from build123d import *

# Parameters (mm, degrees)
BOSS_EXTRUDE4_DEPTH = 4
CUT_EXTRUDE7_DEPTH  = 5
LPATTERN2_COUNT     = 13
LPATTERN2_PITCH     = 9.7389
SKETCH10_W          = 14
SKETCH10_H          = 2.5
BOSS_EXTRUDE5_DEPTH = 115
SKETCH11_R          = 2.5
CUT_EXTRUDE8_DEPTH  = 13


with BuildPart() as part:
    # Sketch9 → Boss-Extrude4 (new body, symmetric)
    with BuildSketch(Plane.XY):
        Polygon((57.5, 6), (49.449989311, 6), (52.64, -0.841), (54.309989311, -0.841), align=None)
        Polygon((52.64, -0.841), (49.449989311, 6), (-57.5, 6), (-57.5, -6), (57.5, -6), (57.5, 6), (54.309989311, -0.841), align=None)
    extrude(amount=BOSS_EXTRUDE4_DEPTH, both=True)

    # Sketch9<4> → Cut-Extrude7 (cut, symmetric)
    with BuildSketch(Plane.XY):
        Polygon((57.5, 6), (49.449989311, 6), (52.64, -0.841), (54.309989311, -0.841), align=None)
    cut_extrude7 = extrude(amount=CUT_EXTRUDE7_DEPTH, both=True, mode=Mode.SUBTRACT)

    # LPattern2: Cut-Extrude7 ×13
    with Locations(*[(-i * LPATTERN2_PITCH, 0, 0) for i in range(1, LPATTERN2_COUNT)]):
        add(cut_extrude7, mode=Mode.SUBTRACT)

    # Sketch10 → Boss-Extrude5 (add)
    with BuildSketch(Plane.ZY.offset(57.5)):
        with Locations((0, -4.75)):
            Rectangle(SKETCH10_W, SKETCH10_H)
    extrude(amount=-BOSS_EXTRUDE5_DEPTH)

    # Sketch11 → Cut-Extrude8 (cut, through all)
    with BuildSketch(Plane.XZ.offset(6)):
        with Locations((-52.5, 0)):
            Circle(SKETCH11_R)
    extrude(amount=-CUT_EXTRUDE8_DEPTH, mode=Mode.SUBTRACT)


solid = part.part
Check sheet for the modelled part. Datum: model origin and axes. Units: mm. A direction names the side the tool comes from. Round coordinates to 2 decimals unless told otherwise and drop trailing zeros. Loops run counter-clockwise (first coordinate to the right, second up) from the corner with the lowest first, then second, coordinate; pieces in that order, holes last. Notation, with made-up numbers: (58.25, 64.5) - (96.25, 64.5) arc R23 ccw to (96.25, 98.5) - close; hole circle Ø8 at (82, 34). An arc over 180 degrees is marked (long way). Answer as CSV lines item,"result". Start each with the question number.
Item 1: Scan lines: line 1 (X direction, y = -1.5, z = 0); line 2 (X direction, y = -1.5, z = 1.5); line 3 (Z direction, x = 51, y = 0.25). Record each from-to range of solid material in increasing order. Write a range as [from, to].
Item 2: Section check A-A (y = 2.25). Count the separate pieces of the cut face and the enclosed holes in it, and give its area (3 significant figures).
Item 3: Section check B-B (x = -42). Record the boundary of the cut face in (y, z).
Item 4: Depth check by flat-ended pin: P1, Ø0.5, axis at x = 53, z = 1.5, coming from the +Y side; P2, Ø6, axis at x = -24.5, z = -1, coming from the +Y side; P3, Ø5, axis at x = 34.5, y = 2, coming from the -Z side; P4, Ø4, axis at x = -52.5, z = 0, coming from the -Y side. Enter the tip coordinate at first touch or a pass-through.
Item 5: Section check C-C (z = 5.25). Record the boundary of the cut face in (x, y).
Item 6: Set-up check for faces 4 (the flat face through (-1, -5, -7)), 5 (the flat face through (-1, 0, -4)), 6 (the flat face through (-26.89, 2.63, 0.06)): record each of +Z, -Z, +X, -X, +Y, -Y from which the full face is reachable in a straight line by a thin tool's end or side.
Item 7: Release check for a two-part mould opening along X. For faces 1 (the flat face through (-1, -5, 7)), 2 (the flat face through (57.5, -1, 0)), 3 (the flat face through (21.806, 2.627, 0.056)) record: +X half, -X half, draft (parallel to the pull), parting line (faces both ways), or undercut.
Report:
1,line 1,"x = [-57.5, -55], [-50, 57.5]"
1,line 2,"x = [-57.5, -54.5], [-50.5, 57.5]"
1,line 3,"z = [-4, 4]"
2,separate pieces,"13"
2,enclosed holes,"0"
2,area,"479 mm2"
3,outline,"(-6, -7) - (-3.5, -7) - (-3.5, -4) - (1.47, -4) - (1.47, 4) - (-3.5, 4) - (-3.5, 7) - (-6, 7) - close"
4,P1,"stops at y = -0.84"
4,P2,"stops at y = 3.94"
4,P3,"stops at z = -4"
4,P4,"passes through"
5,outline,"(-57.5, -6) - (57.5, -6) - (57.5, -3.5) - (-57.5, -3.5) - close"
6,face 4,"-Z, +X, -X, +Y, -Y"
6,face 5,"-Z, +X, -X, +Y"
6,face 6,"+Z, -Z, +Y"
7,face 1,"draft"
7,face 2,"+X half"
7,face 3,"undercut"
